```python
from build123d import *

# Parameters (mm, degrees)
SKETCH1_W           = 33.3
SKETCH1_H           = 20.2
BOSS_EXTRUDE1_DEPTH = 0.508
BOSS_EXTRUDE2_DEPTH = 11.5
BOSS_EXTRUDE2_TAPER = 7
FILLET1_R           = 1.27
FILLET4_R           = 1.27


with BuildPart() as part:
    # Sketch1 → Boss-Extrude1 (new body)
    with BuildSketch(Plane(origin=(0, 0, 0), x_dir=(1, 0, 0), z_dir=(0, 1, 0))):
        Rectangle(SKETCH1_W, SKETCH1_H)
    extrude(amount=BOSS_EXTRUDE1_DEPTH)

    # Sketch2 → Boss-Extrude2 (add)
    with BuildSketch(Plane(origin=(0, 0, 0), x_dir=(1, 0, 0), z_dir=(0, 1, 0))):
        with BuildLine():
            ThreePointArc((-4.875, 7), (-11.875, 0), (-4.875, -7))
            Line((-4.875, -7), (4.875, -7))
            ThreePointArc((4.875, -7), (11.875, 0), (4.875, 7))
            Line((4.875, 7), (-4.875, 7))
        make_face()
    extrude(amount=BOSS_EXTRUDE2_DEPTH, taper=BOSS_EXTRUDE2_TAPER)

    # Fillet1
    fillet1_edges = [part.edges().sort_by_distance(p)[0] for p in [
        (10.46297755, 11.5, 0),
        (0, 11.5, -5.58797755),
        (-10.46297755, 11.5, 0),
        (0, 11.5, 5.58797755),
    ]]
    fillet(fillet1_edges, radius=FILLET1_R)

    # Fillet4
    fillet4_edges = [part.edges().sort_by_distance(p)[0] for p in [
        (11.812625443, 0.508, 0),
        (0, 0.508, -6.937625443),
        (-11.812625443, 0.508, 0),
        (0, 0.508, 6.937625443),
    ]]
    fillet(fillet4_edges, radius=FILLET4_R)


solid = part.part
```
Design review of the part built by this model. Coordinates are the model's own, in mm. A direction names the side the tool comes from. Coordinates: 2 decimals unless noted, no trailing zeros. Loops run counter-clockwise (first coordinate to the right, second up) from the corner with the lowest first, then second, coordinate; pieces in that order, holes last. Notation, with made-up numbers: (28, 14.5) -> (51, 14.5) arc R7 cw to (51, 20.5) -> close; hole circle Ø6 at (-12, 4.5). An arc over 180 degrees is marked (long way). Answer as a JSON object with one key per item and string values.
Q1. Clearance check with flat-ended pins moving along their axes: pin 1 Ø2 at (y, z) = (3.5, -6) entering from -X; pin 2 Ø3 at (y, z) = (9, 4.5) entering from +X; pin 3 Ø3 at (x, y) = (4, 2.5) entering from +Z. State where each tip first meets the part, or that it passes through.
Answer block:
{"pin 1": "stops at x = -9.15", "pin 2": "stops at x = 9.97", "pin 3": "stops at z = 7.06"}
Q2. To check wall thickness, follow L1, parallel to Y at x = 14, z = -0.75; L2, parallel to X at y = 5.5, z = 5; L3, parallel to Z at x = 8, y = 2.25. State the ranges of each line that lie inside material, in increasing order.
Answer block:
{"L1": "y = 0 to 0.51", "L2": "x = -8.75 to 8.75", "L3": "z = -5.95 to 5.95"}
Q3. Take a section at A-A on x = -3.5. Give the boundary of the cut face in (y, z), plus the area to 3 significant figures.
Answer block:
{"outline": "(0, -10.1) -> (0.51, -10.1) -> (0.51, -8.06) arc R1.27 cw to (1.62, -6.8) -> (10.38, -5.72) arc R1.27 ccw to (11.5, -4.46) -> (11.5, 4.46) arc R1.27 ccw to (10.38, 5.72) -> (1.62, 6.8) arc R1.27 cw to (0.51, 8.06) -> (0.51, 10.1) -> (0, 10.1) -> close", "area": "148 mm^2"}
Q4. Tool access review of faces 1 (the cylindrical face through (-0.07, 11.17, -5.32)), 2 (the flat face through (0, 0.508, 9)): name each direction out of +Z, -Z, +X, -X, +Y, -Y from which nothing blocks a thin tool from reaching the whole face with its end or side.
Answer block:
{"face 1": "-Z, +X, -X, +Y", "face 2": "+Y"}
Q5. Take a section at B-B on y = 5. Give the boundary of the cut face in (x, z) (3 decimals).
Answer block:
{"outline": "(-4.875, -6.386) -> (4.875, -6.386) arc R6.386 ccw to (4.875, 6.386) -> (-4.875, 6.386) arc R6.386 ccw to start"}
Q6. Take a section at C-C on y = 9. Give the boundary of the cut face in (x, z) (3 decimals).
Answer block:
{"outline": "(-4.875, -5.895) -> (4.875, -5.895) arc R5.895 ccw to (4.875, 5.895) -> (-4.875, 5.895) arc R5.895 ccw to start"}
